Read the model definition and answer for the solid it produces. Units are mm, in the model's axes. A direction names the side the tool comes from. Round coordinates to 2 decimals unless told otherwise and drop trailing zeros. Loops run counter-clockwise (first coordinate to the right, second up) from the corner with the lowest first, then second, coordinate; pieces in that order, holes last. Notation, with made-up numbers: (62.5, -34.75) - (84.5, -34.75) arc R24 cw to (84.5, -9.75) - close; hole circle Ø6 at (80.25, 8.5). An arc over 180 degrees is marked (long way). Answer as CSV lines item,"result".
```python
from build123d import *

# Parameters (mm, degrees)
SKETCH1_W           = 25.4
SKETCH1_H           = 20.32
BOSS_EXTRUDE1_DEPTH = 1.6
FILLET1_R           = 2
SKETCH2_R           = 1.27
CUT_EXTRUDE1_DEPTH  = 33.567198222
BOSS_EXTRUDE4_START = -0.2
SKETCH5_R           = 1.9
SKETCH5_R_2         = 1.27
BOSS_EXTRUDE4_DEPTH = 2
BOSS_EXTRUDE3_START = 1.6
SKETCH4_W           = 4.5
SKETCH4_H           = 6
BOSS_EXTRUDE3_DEPTH = 1.6


with BuildPart() as part:
    # Sketch1 → Boss-Extrude1 (new body)
    with BuildSketch(Plane.XY):
        with Locations((12.7, 10.16)):
            Rectangle(SKETCH1_W, SKETCH1_H)
    extrude(amount=BOSS_EXTRUDE1_DEPTH)

    # Fillet1
    fillet1_edges = [part.edges().sort_by_distance(p)[0] for p in [
        (0, 20.32, 0.8),
        (25.4, 20.32, 0.8),
        (25.4, 0, 0.8),
        (0, 0, 0.8),
    ]]
    fillet(fillet1_edges, radius=FILLET1_R)

    # Sketch2 → Cut-Extrude1 (cut, through all)
    with BuildSketch(Plane.XY):
        with Locations((2.54, 17.78)):
            Circle(SKETCH2_R)
        with Locations((22.86, 17.78)):
            Circle(SKETCH2_R)
        with Locations((22.86, 2.54)):
            Circle(SKETCH2_R)
        with Locations((2.54, 2.54)):
            Circle(SKETCH2_R)
    extrude(amount=CUT_EXTRUDE1_DEPTH, mode=Mode.SUBTRACT)

    # Sketch5 → Boss-Extrude4 (add)
    # profile 1 of 4: a face of its own
    with BuildSketch(Plane.XY.offset(BOSS_EXTRUDE4_START)):
        with Locations(Location((2.54, 17.78, 0), (0, 0, 180))):
            Circle(SKETCH5_R)
        with Locations((2.54, 17.78)):
            Circle(SKETCH5_R_2, mode=Mode.SUBTRACT)
    # profile 2 of 4: a face of its own
    with BuildSketch(Plane.XY.offset(BOSS_EXTRUDE4_START)):
        with Locations(Location((22.86, 17.78, 0), (0, 0, 180))):
            Circle(SKETCH5_R)
        with Locations((22.86, 17.78)):
            Circle(SKETCH5_R_2, mode=Mode.SUBTRACT)
    # profile 3 of 4: a face of its own
    with BuildSketch(Plane.XY.offset(BOSS_EXTRUDE4_START)):
        with Locations(Location((22.86, 2.54, 0), (0, 0, 180))):
            Circle(SKETCH5_R)
        with Locations((22.86, 2.54)):
            Circle(SKETCH5_R_2, mode=Mode.SUBTRACT)
    # profile 4 of 4: a face of its own
    with BuildSketch(Plane.XY.offset(BOSS_EXTRUDE4_START)):
        with Locations(Location((2.54, 2.54, 0), (0, 0, 180))):
            Circle(SKETCH5_R)
        with Locations((2.54, 2.54)):
            Circle(SKETCH5_R_2, mode=Mode.SUBTRACT)
    extrude(amount=BOSS_EXTRUDE4_DEPTH)

    # Sketch4 → Boss-Extrude3 (add)
    with BuildSketch(Plane.XY.offset(BOSS_EXTRUDE3_START)):
        with Locations((2.45, 10.16)):
            Rectangle(SKETCH4_W, SKETCH4_H)
        with Locations((22.95, 10.16)):
            Rectangle(SKETCH4_W, SKETCH4_H)
    extrude(amount=BOSS_EXTRUDE3_DEPTH)


solid = part.part
```
1) Each of these flat-tipped pins is pushed along its axis until it touches: P1, Ø1.9, axis at x = 22.5, y = 18.5, coming from the +Z side; P2, Ø10, axis at x = 10, y = 6.5, coming from the +Z side; P3, Ø1.3, axis at x = 23.5, z = 2.5, coming from the -Y side. Where does it stop, or does it pass through?
Entries:
P1,"stops at z = 1.8"
P2,"stops at z = 1.6"
P3,"stops at y = 7.16"
2) The mould has two halves that part along X. Classify faces 4 (the face through (1.53, 1.77, 0.79)), 5 (the face through (23, 10, 3.2)), 6 (the face through (25.4, 10, 1)): pulls with the +X half, pulls with the -X half, needs draft (parallel to the pull), parting line crosses it, or undercut.
Entries:
face 4,"undercut"
face 5,"needs draft"
face 6,"pulls with the +X half"
3) Find the intervals of material crossed by line 1 (Y direction, x = 22.86, z = 1.15); line 2 (X direction, y = 7.75, z = 2.3); line 3 (Z direction, x = 11, y = 11.25), in increasing order.
Entries:
line 1,"y = 0 to 1.27, 3.81 to 16.51, 19.05 to 20.32"
line 2,"x = 0.2 to 4.7, 20.7 to 25.2"
line 3,"z = 0 to 1.6"
4) A cutting plane is placed at D-D, the plane z = 1. Determine the outline of the cut face in (x, y).
Entries:
outline,"(0, 2) arc R2 ccw to (2, 0) - (23.4, 0) arc R2 ccw to (25.4, 2) - (25.4, 18.32) arc R2 ccw to (23.4, 20.32) - (2, 20.32) arc R2 ccw to (0, 18.32) - close; hole circle Ø2.54 at (2.54, 2.54); hole circle Ø2.54 at (2.54, 17.78); hole circle Ø2.54 at (22.86, 2.54); hole circle Ø2.54 at (22.86, 17.78)"
5) A cutting plane is placed at A-A, the plane z = 2.8. Determine the outline of the cut face in (x, y), plus the area to 3 significant figures.
Entries:
outline,"(0.2, 7.16) - (4.7, 7.16) - (4.7, 13.16) - (0.2, 13.16) - close; (20.7, 7.16) - (25.2, 7.16) - (25.2, 13.16) - (20.7, 13.16) - close"
area,"54.0 mm^2"
6) A tool of negligible diameter and unlimited length cuts with its end or side. For faces 1 (the face through (25.2, 10, 2)), 2 (the face through (13, 10, 0)), 3 (the face through (13, 20.32, 1)), from which of +Z, -Z, +X, -X, +Y, -Y can it reach the whole face along a straight path? Write none if from no direction.
Entries:
face 1,"+Z, +X, +Y, -Y"
face 2,"-Z"
face 3,"+Z, -Z, +X, -X, +Y"
7) A cutting plane is placed at B-B, the plane y = 2.54. Determine the outline of the cut face in (x, z).
Entries:
outline,"(0, 0) - (0.64, 0) - (0.64, -0.2) - (1.27, -0.2) - (1.27, 1.8) - (0.64, 1.8) - (0.64, 1.6) - (0, 1.6) - close; (3.81, -0.2) - (4.44, -0.2) - (4.44, 0) - (20.96, 0) - (20.96, -0.2) - (21.59, -0.2) - (21.59, 1.8) - (20.96, 1.8) - (20.96, 1.6) - (4.44, 1.6) - (4.44, 1.8) - (3.81, 1.8) - close; (24.13, -0.2) - (24.76, -0.2) - (24.76, 0) - (25.4, 0) - (25.4, 1.6) - (24.76, 1.6) - (24.76, 1.8) - (24.13, 1.8) - close"
8) A cutting plane is placed at C-C, the plane x = 2.54. Count the separate pieces of the cut face and the enclosed holes in it, plus the area to 3 significant figures.
Entries:
separate pieces,"3"
enclosed holes,"0"
area,"35.0 mm^2"
